For this review, take the finished solid that the model builds, in its own axes (mm). Face numbers are marked on the shaded views. Round coordinates to 2 decimals unless told otherwise and drop trailing zeros. Loops run counter-clockwise (first coordinate to the right, second up) from the corner with the lowest first, then second, coordinate; pieces in that order, holes last. Notation, with made-up numbers: M 53.5,52 L 99.5,52 A32 cw 99.5,87 Z; hole C 3.25,10 d8. An arc over 180 degrees is marked long. One line per question, with ' | ' between items. Start each with the question number.
1) We need section D-D (y = -1.75). Give the boundary of the cut face in (x, z), and give its area (3 significant figures).
2) For pin 1 Ø1.5 at (x, y) = (-19, 4) entering from +Z; pin 2 Ø1 at (x, z) = (-19, 0) entering from +Y; pin 3 Ø3 at (x, z) = (-22, 3) entering from +Y, all flat-tipped, find the tip position at first contact; note any pin that passes through.
3) Mouldability with a two-part tool opening along Z and no side actions: class the marked faces 1 and 2 as pulls with the +Z half, pulls with the -Z half, needs draft (parallel to the pull), parting line crosses it, or undercut.
4) For probe 1 along Y at (x, z) = (-21.25, 0); probe 2 along Z at (x, y) = (-26.5, 7.5); probe 3 along Y at (x, z) = (-23.5, -6), list the stretches that pass through material, from the lowest coordinate up. Write a range as from..to.
5) We need section A-A (z = 0). Give the boundary of the cut face in (x, y), and give its area (3 significant figures).
6) We need section C-C (y = 0.5). Give the boundary of the cut face in (x, z), and give its area (3 significant figures).
```python
from build123d import *

# Parameters (mm, degrees)
SKETCH_3_R               = 2
CUT_EXTRUDE_2_DEPTH      = 17
SKETCH_4_W               = 2.5
SKETCH_4_H               = 2.683329606
CUT_EXTRUDE_3_DEPTH      = 17
PATTERN_CIRCULAR_1_COUNT = 15


with BuildPart() as part:
    # 草图1 → 旋转2 (revolve)
    with BuildSketch(Plane.XY, mode=Mode.PRIVATE) as revolve_2_sk:
        Polygon((-27.363734917, 8.847191366), (-27.363734917, 3.847191366), (-28.613734917, 3.847191366), (-28.613734917, 1.847191366), (-16.113734917, 1.847191366), (-16.113734917, 3.847191366), (-17.363734917, 3.847191366), (-17.363734917, 8.847191366), align=None)
    revolve(revolve_2_sk.sketch.rotate(Axis((-48.964491856, 1.847191366, 0), (1, 0, 0)), 90), axis=Axis((-48.964491856, 1.847191366, 0), (1, 0, 0)))

    # 草图3 → 切除-拉伸2 (cut)
    with BuildSketch(Plane.ZY.offset(28.613734917)):
        with Locations((0, 1.847191366)):
            Circle(SKETCH_3_R)
    extrude(amount=-CUT_EXTRUDE_2_DEPTH, mode=Mode.SUBTRACT)

    # 草图4 → 切除-拉伸3 (cut)
    with BuildSketch(Plane.ZY.offset(27.363734917)):
        with Locations((0, 10.188856169)):
            Rectangle(SKETCH_4_W, SKETCH_4_H)
        with BuildLine():
            Line((1.25, 8.847191366), (-1.25, 8.847191366))
            ThreePointArc((-1.25, 8.847191366), (0, 7.597191366), (1.25, 8.847191366))
        make_face()
    cut_extrude_3 = extrude(amount=-CUT_EXTRUDE_3_DEPTH, mode=Mode.SUBTRACT)

    # 阵列(圆周)1: 切除-拉伸3 ×15 about axis
    pattern_circular_1_axis = Axis((0, 1.847191366, 0), (1, 0, 0))
    for i in range(1, PATTERN_CIRCULAR_1_COUNT):
        add(cut_extrude_3.rotate(pattern_circular_1_axis, i * 360 / PATTERN_CIRCULAR_1_COUNT), mode=Mode.SUBTRACT)


solid = part.part
```
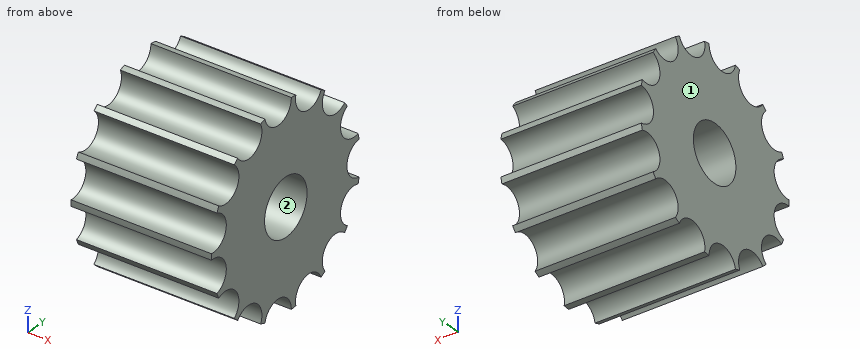
Answers below:
1) outline: M -27.36,-4.82 L -17.36,-4.82 L -17.36,4.82 L -27.36,4.82 Z | area: 96.3 mm^2
2) pin 1: z = 5.67 | pin 2: y = 7.7 | pin 3: y = 8.68
3) face 1: needs draft | face 2: undercut
4) probe 1: -5.15..-0.15, 3.85..7.6 | probe 2: -4.13..-3.85, -1.84..1.84, 3.85..4.13 | probe 3: -0.4..0.32, 1.91..2.95, 5.07..5.45
5) outline: M -27.36,-5.15 L -17.36,-5.15 L -17.36,-0.15 L -27.36,-0.15 Z; M -27.36,3.85 L -17.36,3.85 L -17.36,7.6 L -27.36,7.6 Z | area: 87.5 mm^2
6) outline: M -27.36,-5.87 L -17.36,-5.87 L -17.36,-1.48 L -27.36,-1.48 Z; M -27.36,1.48 L -17.36,1.48 L -17.36,5.87 L -27.36,5.87 Z | area: 87.9 mm^2
